```python
from build123d import *

# Parameters (mm, degrees)
EXTRUDE_1_DEPTH         = 3
SKETCH_2_W              = 11
SKETCH_2_H              = 10
HOLE_WIZARD_16_0_16_1_D = 16
FILLET_1_R              = 0.85


with BuildPart() as part:
    # 草图1 → 凸台-拉伸1 (new body)
    with BuildSketch(Plane.XY.offset(3)):
        with BuildLine():
            Line((7.677617845, 18.755038144), (6.174109651, 19.302270373))
            ThreePointArc((6.174109651, 19.302270373), (5.023989627, 17.932407977), (4.203345275, 16.343118231))
            ThreePointArc((4.203345275, 16.343118231), (2.930312998, 16.618630832), (1.639823102, 16.795136355))
            ThreePointArc((1.639823102, 16.795136355), (1.197968963, 19.299137818), (0, 21.541932676))
            ThreePointArc((0, 21.541932676), (-1.197968963, 19.299137818), (-1.639823102, 16.795136355))
            ThreePointArc((-1.639823102, 16.795136355), (-2.930312998, 16.618630832), (-4.203345275, 16.343118231))
            ThreePointArc((-4.203345275, 16.343118231), (-5.474971289, 18.544986912), (-7.367774901, 20.242795173))
            ThreePointArc((-7.367774901, 20.242795173), (-7.726416477, 17.725527879), (-7.285204612, 15.221413166))
            ThreePointArc((-7.285204612, 15.221413166), (-8.4375, 14.614178689), (-9.539528177, 13.919878849))
            ThreePointArc((-9.539528177, 13.919878849), (-11.4875492, 15.554036889), (-13.846887413, 16.50207782))
            ThreePointArc((-13.846887413, 16.50207782), (-13.322944134, 14.013957677), (-12.051882927, 11.811762904))
            ThreePointArc((-12.051882927, 11.811762904), (-12.926999978, 10.847040913), (-13.725103193, 9.817696642))
            ThreePointArc((-13.725103193, 9.817696642), (-16.114559141, 10.687040464), (-18.655860944, 10.770966338))
            ThreePointArc((-18.655860944, 10.770966338), (-17.312528103, 8.612097355), (-15.364926295, 6.977439714))
            ThreePointArc((-15.364926295, 6.977439714), (-15.857312976, 5.771589919), (-16.255228202, 4.531355326))
            ThreePointArc((-16.255228202, 4.531355326), (-18.797915423, 4.531029235), (-21.214662314, 3.740717353))
            ThreePointArc((-21.214662314, 3.740717353), (-19.213965677, 2.17149099), (-16.824732789, 1.301534317))
            ThreePointArc((-16.824732789, 1.301534317), (-16.875, 0), (-16.824732789, -1.301534317))
            ThreePointArc((-16.824732789, -1.301534317), (-19.213965677, -2.17149099), (-21.214662314, -3.740717353))
            ThreePointArc((-21.214662314, -3.740717353), (-18.797915423, -4.531029235), (-16.255228202, -4.531355326))
            ThreePointArc((-16.255228202, -4.531355326), (-15.857312976, -5.771589919), (-15.364926295, -6.977439714))
            ThreePointArc((-15.364926295, -6.977439714), (-17.312528103, -8.612097355), (-18.655860944, -10.770966338))
            ThreePointArc((-18.655860944, -10.770966338), (-16.114559141, -10.687040464), (-13.725103193, -9.817696642))
            ThreePointArc((-13.725103193, -9.817696642), (-12.926999978, -10.847040913), (-12.051882927, -11.811762904))
            ThreePointArc((-12.051882927, -11.811762904), (-13.322944134, -14.013957677), (-13.846887413, -16.50207782))
            ThreePointArc((-13.846887413, -16.50207782), (-11.4875492, -15.554036889), (-9.539528177, -13.919878849))
            ThreePointArc((-9.539528177, -13.919878849), (-8.4375, -14.614178689), (-7.285204612, -15.221413166))
            ThreePointArc((-7.285204612, -15.221413166), (-7.726416477, -17.725527879), (-7.367774901, -20.242795173))
            ThreePointArc((-7.367774901, -20.242795173), (-5.474971289, -18.544986912), (-4.203345275, -16.343118231))
            ThreePointArc((-4.203345275, -16.343118231), (-2.930312998, -16.618630832), (-1.639823102, -16.795136355))
            ThreePointArc((-1.639823102, -16.795136355), (-1.197968963, -19.299137818), (0, -21.541932676))
            ThreePointArc((0, -21.541932676), (1.197968963, -19.299137818), (1.639823102, -16.795136355))
            ThreePointArc((1.639823102, -16.795136355), (2.930312998, -16.618630832), (4.203345275, -16.343118231))
            ThreePointArc((4.203345275, -16.343118231), (5.023989627, -17.932407977), (6.174109651, -19.302270373))
            Line((6.174109651, -19.302270373), (7.677617845, -18.755038144))
            ThreePointArc((7.677617845, -18.755038144), (7.678130324, -16.966379766), (7.285204612, -15.221413166))
            ThreePointArc((7.285204612, -15.221413166), (8.4375, -14.614178689), (9.539528177, -13.919878849))
            ThreePointArc((9.539528177, -13.919878849), (11.4875492, -15.554036889), (13.846887413, -16.50207782))
            ThreePointArc((13.846887413, -16.50207782), (13.322944134, -14.013957677), (12.051882927, -11.811762904))
            ThreePointArc((12.051882927, -11.811762904), (12.926999978, -10.847040913), (13.725103193, -9.817696642))
            ThreePointArc((13.725103193, -9.817696642), (16.114559141, -10.687040464), (18.655860944, -10.770966338))
            ThreePointArc((18.655860944, -10.770966338), (17.312528103, -8.612097355), (15.364926295, -6.977439714))
            ThreePointArc((15.364926295, -6.977439714), (15.857312976, -5.771589919), (16.255228202, -4.531355326))
            ThreePointArc((16.255228202, -4.531355326), (18.797915423, -4.531029235), (21.214662314, -3.740717353))
            ThreePointArc((21.214662314, -3.740717353), (19.213965677, -2.17149099), (16.824732789, -1.301534317))
            ThreePointArc((16.824732789, -1.301534317), (16.875, 0), (16.824732789, 1.301534317))
            ThreePointArc((16.824732789, 1.301534317), (19.213965677, 2.17149099), (21.214662314, 3.740717353))
            ThreePointArc((21.214662314, 3.740717353), (18.797915423, 4.531029235), (16.255228202, 4.531355326))
            ThreePointArc((16.255228202, 4.531355326), (15.857312976, 5.771589919), (15.364926295, 6.977439714))
            ThreePointArc((15.364926295, 6.977439714), (17.312528103, 8.612097355), (18.655860944, 10.770966338))
            ThreePointArc((18.655860944, 10.770966338), (16.114559141, 10.687040464), (13.725103193, 9.817696642))
            ThreePointArc((13.725103193, 9.817696642), (12.926999978, 10.847040913), (12.051882927, 11.811762904))
            ThreePointArc((12.051882927, 11.811762904), (13.322944134, 14.013957677), (13.846887413, 16.50207782))
            ThreePointArc((13.846887413, 16.50207782), (11.4875492, 15.554036889), (9.539528177, 13.919878849))
            ThreePointArc((9.539528177, 13.919878849), (8.4375, 14.614178689), (7.285204612, 15.221413166))
            ThreePointArc((7.285204612, 15.221413166), (7.678130324, 16.966379766), (7.677617845, 18.755038144))
        make_face()
    extrude(amount=-EXTRUDE_1_DEPTH)

    # 草图2 → 旋转1 (revolve)
    with BuildSketch(Plane(origin=(0, 0, 0), x_dir=(1, 0, 0), z_dir=(0, 1, 0))):
        with Locations((5.5, -8)):
            Rectangle(SKETCH_2_W, SKETCH_2_H)
    revolve(axis=Axis((0, 0, 3), (0, 0, 1)))

    # Ø16.0 (16) 直径孔1 (through all)
    with Locations(Plane(origin=(0, 0, 0), x_dir=(-1, 0, 0), z_dir=(0, 0, -1))):
        with Locations((0, 0)):
            Hole(HOLE_WIZARD_16_0_16_1_D / 2)

    # 倒角1
    # the kernel refuses this chamfer: 2.4092894, 1.801151222 mm, written as the material it takes off along each edge
    with BuildSketch(Plane(origin=(21.214662314, 3.740717353, 8.457999089), x_dir=(-0.9419139002762257, 0.33585443940259097, 0), z_dir=(0, 0, -1)), Plane(origin=(21.214662314, -3.740717353, 8.457999089), x_dir=(-0.7702405580042077, 0.6377534655377162, 0), z_dir=(0, 0, -1)), Plane(origin=(18.655860944, -10.770966338, 8.457999089), x_dir=(-0.5056648368969275, 0.8627300114902714, 0), z_dir=(0, 0, -1)), Plane(origin=(13.846887413, -16.50207782, 8.457999089), x_dir=(-0.18009847364168569, 0.9836485855181895, 0), z_dir=(0, 0, -1)), Plane(origin=(0, -21.541932676, 8.457999089), x_dir=(0.4943136881093548, 0.8692836002983879, 0), z_dir=(0, 0, -1)), Plane(origin=(-7.367774901, -20.242795173, 8.457999089), x_dir=(0.7618154266345339, 0.6477941461156027, 0), z_dir=(0, 0, -1)), Plane(origin=(-13.846887413, -16.50207782, 8.457999089), x_dir=(0.9374309815093264, 0.3481711574878957, 0), z_dir=(0, 0, -1)), Plane(origin=(18.655860944, 10.770966338, 8.457999089), x_dir=(-0.9999785250062793, -0.00655358880811246, 0), z_dir=(0, 0, -1))) as chamfer_1_piece_1:
        with BuildLine():
            Line((2.119488029, 0), (0.84248532, -1.499732591))
            ThreePointArc((0.84248532, -1.499732591), (0.389416714, -0.786885265), (0, 0))
            ThreePointArc((0, 0), (1.091111326, 0.069719636), (2.119488029, 0))
        make_face()
    extrude(amount=13.915998179, mode=Mode.SUBTRACT)
    with BuildSketch(Plane(origin=(-18.655860944, -10.770966338, 8.457999089), x_dir=(0.48404481309239716, 0.8750432097435796, 0), z_dir=(0, 0, -1)), Plane(origin=(-21.214662314, -3.740717353, 8.457999089), x_dir=(0.7541357430052743, 0.6567185707149471, 0), z_dir=(0, 0, -1)), Plane(origin=(-21.214662314, 3.740717353, 8.457999089), x_dir=(0.9332667724535083, 0.35918397992423245, 0), z_dir=(0, 0, -1)), Plane(origin=(-18.655860944, 10.770966338, 8.457999089), x_dir=(0.9998320555932133, 0.01832650016368515, 0), z_dir=(0, 0, -1)), Plane(origin=(-13.846887413, 16.50207782, 8.457999089), x_dir=(0.9458028368787899, -0.32474142598694317, 0), z_dir=(0, 0, -1)), Plane(origin=(-7.367774901, 20.242795173, 8.457999089), x_dir=(0.777695837473541, -0.6286407434905311, 0), z_dir=(0, 0, -1)), Plane(origin=(0, 21.541932676, 8.457999089), x_dir=(0.5157872425008245, -0.8567167095798913, 0), z_dir=(0, 0, -1)), Plane(origin=(13.846887413, 16.50207782, 8.457999089), x_dir=(-0.15557093497995983, -0.9878247234147671, 0), z_dir=(0, 0, -1))) as chamfer_1_piece_2:
        with BuildLine():
            Line((1.72016841, 0), (1.038059727, 1.847880275))
            ThreePointArc((1.038059727, 1.847880275), (0.473607386, 0.985434319), (0, 0))
            ThreePointArc((0, 0), (0.87677191, -0.045878267), (1.72016841, 0))
        make_face()
    extrude(amount=13.915998179, mode=Mode.SUBTRACT)

    # 圆角1
    fillet_1_edges = [part.edges().sort_by_distance(p)[0] for p in [
        (16.824732789, 1.301534317, 1.5),
        (16.824732789, -1.301534317, 1.5),
        (16.255228202, -4.531355326, 1.5),
        (15.364926295, -6.977439714, 1.5),
        (13.725103193, -9.817696642, 1.5),
        (12.051882927, -11.811762904, 1.5),
        (9.539528177, -13.919878849, 1.5),
        (7.285204612, -15.221413166, 1.5),
        (4.203345275, -16.343118231, 1.5),
        (1.639823102, -16.795136355, 1.5),
        (-1.639823102, -16.795136355, 1.5),
        (-4.203345275, -16.343118231, 1.5),
        (-7.285204612, -15.221413166, 1.5),
        (-9.539528177, -13.919878849, 1.5),
        (-12.051882927, -11.811762904, 1.5),
        (-13.725103193, -9.817696642, 1.5),
        (-15.364926295, -6.977439714, 1.5),
        (-16.255228202, -4.531355326, 1.5),
        (-16.824732789, -1.301534317, 1.5),
        (-16.824732789, 1.301534317, 1.5),
        (-16.255228202, 4.531355326, 1.5),
        (-15.364926295, 6.977439714, 1.5),
        (-13.725103193, 9.817696642, 1.5),
        (-12.051882927, 11.811762904, 1.5),
        (-9.539528177, 13.919878849, 1.5),
        (-7.285204612, 15.221413166, 1.5),
        (-4.203345275, 16.343118231, 1.5),
        (-1.639823102, 16.795136355, 1.5),
        (1.639823102, 16.795136355, 1.5),
        (4.203345275, 16.343118231, 1.5),
        (7.285204612, 15.221413166, 1.5),
        (9.539528177, 13.919878849, 1.5),
        (12.051882927, 11.811762904, 1.5),
        (13.725103193, 9.817696642, 1.5),
        (15.364926295, 6.977439714, 1.5),
        (16.255228202, 4.531355326, 1.5),
    ]]
    fillet(fillet_1_edges, radius=FILLET_1_R)


solid = part.part
```
The listing builds one solid part. Answer for the finished solid, in the listing's coordinates (mm). A direction names the side the tool comes from. Give positions to 0.01 mm unless a question says otherwise; leave off trailing zeros. Loops run counter-clockwise (first coordinate to the right, second up) from the corner with the lowest first, then second, coordinate; pieces in that order, holes last. Notation, with made-up numbers: (-26.75, 49) - (14.25, 49) arc R24 cw to (14.25, 71) - close; hole circle Ø1 at (57.25, 62.25). An arc over 180 degrees is marked (long way). Answer as CSV lines item,"result". Start each with the question number.
Item 1: Each of these flat-tipped pins is pushed along its axis until it touches: pin 1 (1.5 mm diameter, centred on x = 6.5, y = 10, fed in from +Z); pin 2 (2 mm diameter, centred on y = 10.5, z = 9.5, fed in from -X); pin 3 (6 mm diameter, centred on x = -8.5, z = 3.5, fed in from +Y). Where does it stop, or does it pass through?
Item 2: A cutting plane is placed at B-B on x = 0. Determine the outline of the cut face in (y, z).
Item 3: For faces 1 (the face through (11.03, -15.26, 1.52)), 2 (the face through (16.875, -0.009, 1.521)), 3 (the face through (12.922, -10.854, 1.521)), determine the directions among +Z, -Z, +X, -X, +Y, -Y from which every point of the face is accessible in a straight line to the end or side of a thin tool.
Item 4: A cutting plane is placed at D-D on y = -13. Determine the outline of the cut face in (x, z).
Item 5: The mould has two halves that part along Y. Classify faces 4 (the face through (-6.864, 18.664, 1.521)), 5 (the face through (2.92, -16.62, 1.52)), 6 (the face through (-13.11, -13.51, 1.52)): +Y half, -Y half, draft (parallel to the pull), parting line (faces both ways), or undercut.
Item 6: Find the intervals of material crossed by line 1 (X direction, y = -15, z = 1.5); line 2 (Y direction, x = 0, z = 5); line 3 (Z direction, x = 13.5, y = 6), in increasing order. Write a range as from..to.
Item 7: A cutting plane is placed at A-A on y = 0. Determine the outline of the cut face in (x, z) (3 decimals), then the cut area to 3 significant figures.
Item 8: A cutting plane is placed at C-C on z = 4.75. Determine the outline of the cut face in (x, y).
Found:
1,pin 1,"stops at z = 3"
1,pin 2,"stops at x = -5.55"
1,pin 3,"stops at y = 19.16"
2,outline,"(-19.9, 0) - (-8, 0) - (-8, 13) - (-11, 13) - (-11, 3) - (-19.9, 3) - close; (8, 0) - (19.9, 0) - (19.9, 3) - (11, 3) - (11, 13) - (8, 13) - close"
3,face 1,"+Z, -Z, -Y"
3,face 2,"+Z, -Z, +X"
3,face 3,"+Z, -Z"
4,outline,"(-12.85, 0) - (12.85, 0) - (12.85, 3) - (-12.85, 3) - close"
5,face 4,"+Y half"
5,face 5,"-Y half"
5,face 6,"undercut"
6,line 1,"x = -13.23..-10.68, -7.77..7.77, 10.68..12.99"
6,line 2,"y = -11..-8, 8..11"
6,line 3,"z = 0..3"
7,outline,"(-16.875, 0) - (-8, 0) - (-8, 13) - (-11, 13) - (-11, 3) - (-16.875, 3) - close; (8, 0) - (16.875, 0) - (16.875, 3) - (11, 3) - (11, 13) - (8, 13) - close"
7,area,"113 mm^2"
8,outline,"circle Ø22 at (0, 0); hole circle Ø16 at (0, 0)"
